Geometry: final body of the model. Coordinates: model frame, mm. A direction names the side the tool comes from. Coordinates: 2 decimals unless noted, no trailing zeros. Order: outer loops, then holes, each group sorted by start corner. A loop starts at its lowest first (then second) coordinate and runs counter-clockwise, first axis right, second up. Notation, with made-up numbers: (51, 30.5) -> (67, 30.5) arc R12 cw to (67, 53.5) -> close; hole circle Ø4 at (1, -37.75). An arc over 180 degrees is marked (long way). Use CSV: the item, a comma, the result in double quotes. Start each with the question number.
from build123d import *

# Parameters (mm, degrees)
SKETCH1_R                      = 21.2725
BOSS_EXTRUDE1_DEPTH            = 3.175
SKETCH2_R                      = 15.875
BOSS_EXTRUDE2_DEPTH            = 9.525
F_3_16_0_1875_DIAMETER_HOLE1_D = 4.7625
F_2_56_TAPPED_HOLE3_D          = 1.778
CIRPATTERN1_COUNT              = 3
F_8_32_TAPPED_HOLE1_D          = 3.4544
F_8_32_TAPPED_HOLE1_DEPTH      = 21.2715
F_8_32_TAPPED_HOLE1_TIP        = 1.037806461
SKETCH14_R                     = 7.9375
CUT_EXTRUDE1_DEPTH             = 3.8862


with BuildPart() as part:
    # Sketch1 → Boss-Extrude1 (new body)
    with BuildSketch(Plane.XY):
        Circle(SKETCH1_R)
    extrude(amount=BOSS_EXTRUDE1_DEPTH)

    # Sketch2 → Boss-Extrude2 (add)
    with BuildSketch(Plane.XY.offset(3.175)):
        with Locations(Location((0, 0, 0), (0, 0, 180))):
            Circle(SKETCH2_R)
    extrude(amount=BOSS_EXTRUDE2_DEPTH)

    # 3/16 (0.1875) Diameter Hole1 (through all)
    with Locations(Plane.XY.offset(12.7)):
        with Locations((0, 0)):
            Hole(F_3_16_0_1875_DIAMETER_HOLE1_D / 2)

    # #2-56 Tapped Hole3 (through all)
    with Locations(Plane.XY.offset(3.175)):
        with Locations((0, 19.05)):
            f_2_56_tapped_hole3 = Hole(F_2_56_TAPPED_HOLE3_D / 2)

    # CirPattern1: #2-56 Tapped Hole3 ×3 about axis
    cirpattern1_axis = Axis((0, 0, 0), (0, 0, 1))
    for i in range(1, CIRPATTERN1_COUNT):
        add(f_2_56_tapped_hole3.rotate(cirpattern1_axis, i * 360 / CIRPATTERN1_COUNT), mode=Mode.SUBTRACT)

    # #8-32 Tapped Hole1
    with Locations(Plane.XZ.offset(21.2725)):
        with Locations((0, 7.9248)):
            Hole(F_8_32_TAPPED_HOLE1_D / 2, depth=F_8_32_TAPPED_HOLE1_DEPTH)
            with Locations((0, 0, -(F_8_32_TAPPED_HOLE1_DEPTH + F_8_32_TAPPED_HOLE1_TIP / 2))):  # 118° drill point
                Cone(0, F_8_32_TAPPED_HOLE1_D / 2, F_8_32_TAPPED_HOLE1_TIP, mode=Mode.SUBTRACT)

    # Sketch14 → Cut-Extrude1 (cut)
    with BuildSketch(Plane(origin=(0, 0, 0), x_dir=(-1, 0, 0), z_dir=(0, 0, -1))):
        Circle(SKETCH14_R)
    extrude(amount=-CUT_EXTRUDE1_DEPTH, mode=Mode.SUBTRACT)


solid = part.part
(1) Access query for faces 4 (the face through (0.31, 2.36, 8.23)), 5 (the face through (-2, 2, 3.886)), 6 (the face through (-3, -16, 3.175)), 7 (the face through (-1.595, -8.659, 7.263)). Directions: +Z, -Z, +X, -X, +Y, -Y. A direction counts if a zero-diameter tool reaches every point of the face in a straight line with its end or side. Return the directions, or none.
(2) Line query: line 1 (Y direction, x = 0, z = 2.5); line 2 (Y direction, x = 0, z = 11) (3 decimals); line 3 (Z direction, x = -1, y = -3). Output: solid intervals per line, ascending. Write a range as from..to.
(3) Section C-C (y = -5). Return loops of the section in (x, z) (3 decimals), then the cut area to 3 significant figures.
(4) Section D-D (z = 2.25). State how many separate pieces and enclosed holes the cut face has, then the cut area to 3 significant figures.
(5) Section B-B (x = 0). Return loops of the section in (y, z) (1 decimal), then the cut area to 3 significant figures.
(6) Section A-A (y = 0). Return loops of the section in (x, z) (1 decimal).
(7) First-contact query: pin 1 (8 mm diameter, centred on x = 0, y = 3.5, fed in from -Z); pin 2 (1.4 mm diameter, centred on x = 0, y = 19.05, fed in from +Z); pin 3 (2 mm diameter, centred on x = -1.5, z = 4, fed in from -Y); pin 4 (1 mm diameter, centred on y = -0.5, z = 5.5, fed in from +X) (3 decimals). Flat tips, straight axial feed; report the tip coordinate or a pass-through.
(8) Mould query, pull axis Y, two halves, no side actions, for faces 1 (the face through (-3, 0, 12.7)), 2 (the face through (0.655, 19.651, 1.565)), 3 (the face through (3.441, 15.497, 7.871)). Classes: pulls with the +Y half, pulls with the -Y half, needs draft (parallel to the pull), parting line crosses it, or undercut.
Check sheet entries:
1,face 4,"+Z, -Z"
1,face 5,"-Z"
1,face 6,"+Z"
1,face 7,"-Y"
2,line 1,"y = -21.27..-7.94, 7.94..18.16, 19.94..21.27"
2,line 2,"y = -15.875..-2.381, 2.381..15.875"
2,line 3,"z = 3.89..6.52, 9.33..12.7"
3,outline,"(-20.677, 0) -> (-6.165, 0) -> (-6.165, 3.886) -> (6.165, 3.886) -> (6.165, 0) -> (20.677, 0) -> (20.677, 3.175) -> (15.067, 3.175) -> (15.067, 12.7) -> (-15.067, 12.7) -> (-15.067, 3.175) -> (-20.677, 3.175) -> close; hole circle Ø3.454 at (0, 7.925)"
3,area,"361 mm^2"
4,separate pieces,"1"
4,enclosed holes,"4"
4,area,"1,220 mm^2"
5,outline,"(-21.3, 0) -> (-7.9, 0) -> (-7.9, 3.9) -> (-2.4, 3.9) -> (-2.4, 6.2) -> (-15.9, 6.2) -> (-15.9, 3.2) -> (-21.3, 3.2) -> close; (-15.9, 9.7) -> (-2.4, 9.7) -> (-2.4, 12.7) -> (-15.9, 12.7) -> close; (2.4, 3.9) -> (7.9, 3.9) -> (7.9, 0) -> (18.2, 0) -> (18.2, 3.2) -> (15.9, 3.2) -> (15.9, 12.7) -> (2.4, 12.7) -> close; (19.9, 0) -> (21.3, 0) -> (21.3, 3.2) -> (19.9, 3.2) -> close"
5,area,"282 mm^2"
6,outline,"(-21.3, 0) -> (-7.9, 0) -> (-7.9, 3.9) -> (-2.4, 3.9) -> (-2.4, 12.7) -> (-15.9, 12.7) -> (-15.9, 3.2) -> (-21.3, 3.2) -> close; (2.4, 3.9) -> (7.9, 3.9) -> (7.9, 0) -> (21.3, 0) -> (21.3, 3.2) -> (15.9, 3.2) -> (15.9, 12.7) -> (2.4, 12.7) -> close"
7,pin 1,"stops at z = 3.89"
7,pin 2,"passes through"
7,pin 3,"stops at y = -21.25"
7,pin 4,"stops at x = 15.875"
8,face 1,"needs draft"
8,face 2,"undercut"
8,face 3,"parting line crosses it"
